Part print with two shaded views. Sizes in mm from the minimum x, y, z corner. A direction names the side the tool comes from. Round coordinates to 2 decimals unless told otherwise and drop trailing zeros. Order: outer loops, then holes, each group sorted by start corner. A loop starts at its lowest first (then second) coordinate and runs counter-clockwise, first axis right, second up. Notation, with made-up numbers: (42.25, -31) - (61.25, -31) arc R18 ccw to (61.25, -5) - close; hole circle Ø7 at (-13, 8). An arc over 180 degrees is marked (long way). Answer as CSV lines item,"result". Start each with the question number.
1. Pin check, flat tip, straight feed: pin 1 Ø1 at (x, z) = (73.5, 58) entering from -Y. Stop position of the tip, or through.
2. Band-saw the part on B-B on z = 110.5. List the corners of the cut face in (x, y), then the cut area to 3 significant figures.
3. Pull direction X, two halves, no side cores. Call the marked faces 3, 4 and 5: released by +X, released by -X, zero draft, split by the parting line, or undercut.
4. Band-saw the part on C-C on x = 107. List the corners of the cut face in (y, z), then the cut area to 3 significant figures.
5. Band-saw the part on A-A on y = 14. List the corners of the cut face in (x, z).
6. 3-axis set-ups, long thin cutter, end or side, ignore diameter. For the marked faces 1 and 2: which of +Z, -Z, +X, -X, +Y, -Y reach the whole face in a straight line?
7. Wall check: line 1 along X through (y, z) = (44, 130); line 2 along Y through (x, z) = (25, 90); line 3 along Y through (x, z) = (9.5, 188). Give the ranges that are in metal, low to high. Write a range as [from, to].
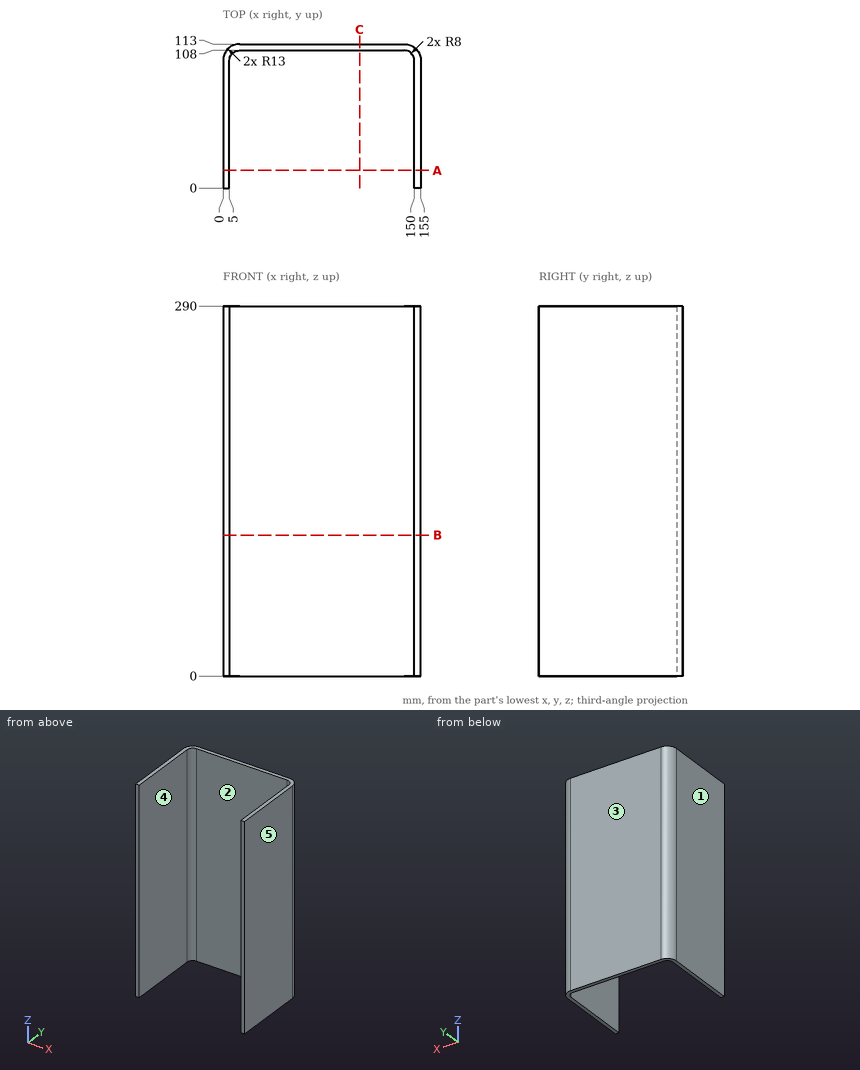
Reply:
1,pin 1,"stops at y = 108"
2,outline,"(0, 0) - (5, 0) - (5, 100) arc R8 cw to (13, 108) - (142, 108) arc R8 cw to (150, 100) - (150, 0) - (155, 0) - (155, 100) arc R13 ccw to (142, 113) - (13, 113) arc R13 ccw to (0, 100) - close"
2,area,"1,810 mm2"
3,face 3,"zero draft"
3,face 4,"undercut"
3,face 5,"released by +X"
4,outline,"(108, 0) - (113, 0) - (113, 290) - (108, 290) - close"
4,area,"1,450 mm2"
5,outline,"(0, 0) - (5, 0) - (5, 290) - (0, 290) - close; (150, 0) - (155, 0) - (155, 290) - (150, 290) - close"
6,face 1,"+Z, -Z, -X, +Y, -Y"
6,face 2,"+Z, -Z, -Y"
7,line 1,"x = [0, 5], [150, 155]"
7,line 2,"y = [108, 113]"
7,line 3,"y = [107.19, 112.52]"
